Geometry: see drawing. Coordinates: mm, zero at the bounding-box minimum. A direction names the side the tool comes from. Round coordinates to 2 decimals unless told otherwise and drop trailing zeros. Order: outer loops, then holes, each group sorted by start corner. A loop starts at its lowest first (then second) coordinate and runs counter-clockwise, first axis right, second up. Notation, with made-up numbers: (-16.5, 44) -> (4.5, 44) arc R20 cw to (4.5, 64) -> close; hole circle Ø9 at (69, 36). An arc over 180 degrees is marked (long way). Use a Markdown table: item, result.
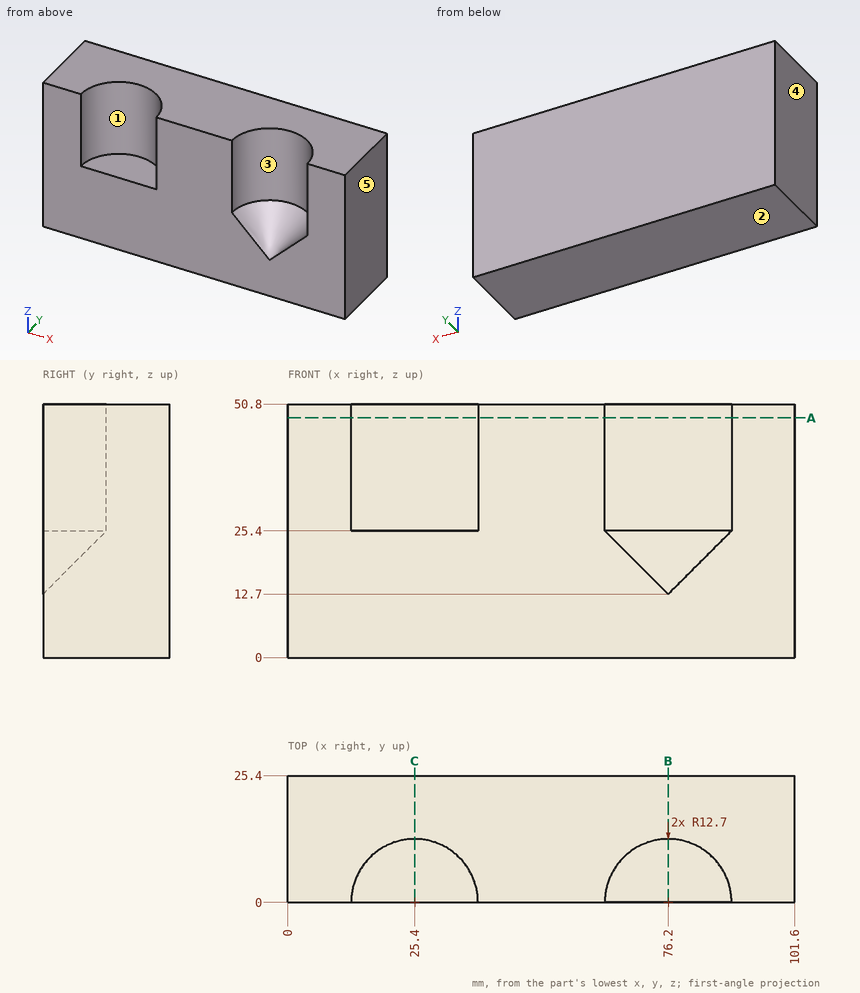
1) Cut plane C-C on x = 25.4. Return loops of the section in (y, z), and give its area (3 significant figures).
Answer key:
| item | result |
|---|---|
| outline | (0, 0) -> (25.4, 0) -> (25.4, 50.8) -> (12.7, 50.8) -> (12.7, 25.4) -> (0, 25.4) -> close |
| area | 968 mm^2 |
2) Contact query for flat-ended pins moving along their axis: P1, Ø4, axis at x = 24.5, y = 6.5, coming from the +Z side; P2, Ø1, axis at x = 68, z = 24.5, coming from the -Y side. Output: stop coordinate, or through.
Answer key:
| item | result |
|---|---|
| P1 | stops at z = 25.4 |
| P2 | stops at y = 7.6 |
3) Ray query, probe 1 along X at (y, z) = (10, 45); probe 2 along X at (y, z) = (5.25, 27); probe 3 along Y at (x, z) = (26.5, 26.5). Return the intervals inside material, ascending.
Answer key:
| item | result |
|---|---|
| probe 1 | x = 0 to 17.57, 33.23 to 68.37, 84.03 to 101.6 |
| probe 2 | x = 0 to 13.84, 36.96 to 64.64, 87.76 to 101.6 |
| probe 3 | y = 12.65 to 25.4 |
4) Set-up query: the marked faces 1 and 2. Return all of +Z, -Z, +X, -X, +Y, -Y with unobstructed straight access to the full face (end or side cutting, diameter ignored); none if empty.
Answer key:
| item | result |
|---|---|
| face 1 | +Z, -Y |
| face 2 | -Z, +X, -X, +Y, -Y |
5) Cut plane B-B on x = 76.2. Return loops of the section in (y, z).
Answer key:
| item | result |
|---|---|
| outline | (0, 0) -> (25.4, 0) -> (25.4, 50.8) -> (12.7, 50.8) -> (12.7, 25.4) -> (0, 12.7) -> close |
6) Draft query along X for the marked faces 3, 4 and 5. Return one class per face: released by +X, released by -X, zero draft, split by the parting line, or undercut.
Answer key:
| item | result |
|---|---|
| face 3 | undercut |
| face 4 | released by -X |
| face 5 | released by +X |
7) Cut plane A-A on z = 48. Return loops of the section in (x, y).
Answer key:
| item | result |
|---|---|
| outline | (0, 0) -> (12.7, 0) arc R12.7 cw to (38.1, 0) -> (63.5, 0) arc R12.7 cw to (88.9, 0) -> (101.6, 0) -> (101.6, 25.4) -> (0, 25.4) -> close |
